```python
from build123d import *

# Parameters (mm, degrees)
BOSS_EXTRUDE1_DEPTH = 30
CUT_EXTRUDE2_REACH  = 61.852
SKETCH3_R           = 2
SKETCH3_R_2         = 6
FILLET1_R           = 1


with BuildPart() as part:
    # Sketch2 → Boss-Extrude1 (new body)
    with BuildSketch(Plane(origin=(0, 0, 0), x_dir=(1, 0, 0), z_dir=(0, 1, 0))):
        with BuildLine():
            Line((0, 50), (13.5, 50))
            Line((13.5, 50), (13.5, 0))
            Line((13.5, 0), (8.5, 0))
            Line((8.5, 0), (8.5, 25))
            ThreePointArc((8.5, 25), (7.621320344, 27.121320344), (5.5, 28))
            Line((5.5, 28), (0, 28))
            Line((0, 28), (0, 33))
            ThreePointArc((0, 33), (6, 39), (0, 45))
            Line((0, 45), (0, 50))
        make_face()
    extrude(amount=BOSS_EXTRUDE1_DEPTH)

    # Sketch3 → Cut-Extrude2 (cut, up to next)
    with BuildSketch(Plane(origin=(13.5, 0, 0), x_dir=(0, 0, -1), z_dir=(1, 0, 0)), mode=Mode.PRIVATE) as cut_extrude2_sk1:
        with BuildLine():
            ThreePointArc((0, 15), (3.514718626, 23.485281374), (12, 27))
            Line((12, 27), (22, 30))
            Line((22, 30), (0, 30))
            Line((0, 30), (0, 15))
        make_face()
    cut_extrude2_tool1 = extrude(cut_extrude2_sk1.sketch, amount=-CUT_EXTRUDE2_REACH, mode=Mode.PRIVATE) & part.part
    # Sketch3 → Cut-Extrude2 (cut, up to next)
    with BuildSketch(Plane(origin=(13.5, 0, 0), x_dir=(0, 0, -1), z_dir=(1, 0, 0)), mode=Mode.PRIVATE) as cut_extrude2_sk2:
        with BuildLine():
            ThreePointArc((12, 3), (3.514718626, 6.514718626), (0, 15))
            Line((0, 15), (0, 0))
            Line((0, 0), (22, 0))
            Line((22, 0), (12, 3))
        make_face()
    cut_extrude2_tool2 = extrude(cut_extrude2_sk2.sketch, amount=-CUT_EXTRUDE2_REACH, mode=Mode.PRIVATE) & part.part
    # Sketch3 → Cut-Extrude2 (cut, up to next)
    with BuildSketch(Plane(origin=(13.5, 0, 0), x_dir=(0, 0, -1), z_dir=(1, 0, 0)), mode=Mode.PRIVATE) as cut_extrude2_sk3:
        with Locations((30.5, 5)):
            Circle(SKETCH3_R)
    cut_extrude2_tool3 = extrude(cut_extrude2_sk3.sketch, amount=-CUT_EXTRUDE2_REACH, mode=Mode.PRIVATE) & part.part
    # Sketch3 → Cut-Extrude2 (cut, up to next)
    with BuildSketch(Plane(origin=(13.5, 0, 0), x_dir=(0, 0, -1), z_dir=(1, 0, 0)), mode=Mode.PRIVATE) as cut_extrude2_sk4:
        with Locations((47.5, 5)):
            Circle(SKETCH3_R)
    cut_extrude2_tool4 = extrude(cut_extrude2_sk4.sketch, amount=-CUT_EXTRUDE2_REACH, mode=Mode.PRIVATE) & part.part
    # Sketch3 → Cut-Extrude2 (cut, up to next)
    with BuildSketch(Plane(origin=(13.5, 0, 0), x_dir=(0, 0, -1), z_dir=(1, 0, 0)), mode=Mode.PRIVATE) as cut_extrude2_sk5:
        with Locations((47.5, 5)):
            Circle(SKETCH3_R)
    cut_extrude2_tool5 = extrude(cut_extrude2_sk5.sketch, amount=-CUT_EXTRUDE2_REACH, mode=Mode.PRIVATE) & part.part
    # Sketch3 → Cut-Extrude2 (cut, up to next)
    with BuildSketch(Plane(origin=(13.5, 0, 0), x_dir=(0, 0, -1), z_dir=(1, 0, 0)), mode=Mode.PRIVATE) as cut_extrude2_sk6:
        with Locations((12, 15)):
            Circle(SKETCH3_R_2)
    cut_extrude2_tool6 = extrude(cut_extrude2_sk6.sketch, amount=-CUT_EXTRUDE2_REACH, mode=Mode.PRIVATE) & part.part
    # Sketch3 → Cut-Extrude2 (cut, up to next)
    with BuildSketch(Plane(origin=(13.5, 0, 0), x_dir=(0, 0, -1), z_dir=(1, 0, 0)), mode=Mode.PRIVATE) as cut_extrude2_sk7:
        with Locations((30.5, 25)):
            Circle(SKETCH3_R)
    cut_extrude2_tool7 = extrude(cut_extrude2_sk7.sketch, amount=-CUT_EXTRUDE2_REACH, mode=Mode.PRIVATE) & part.part
    # Sketch3 → Cut-Extrude2 (cut, up to next)
    with BuildSketch(Plane(origin=(13.5, 0, 0), x_dir=(0, 0, -1), z_dir=(1, 0, 0)), mode=Mode.PRIVATE) as cut_extrude2_sk8:
        with Locations((47.5, 25)):
            Circle(SKETCH3_R)
    cut_extrude2_tool8 = extrude(cut_extrude2_sk8.sketch, amount=-CUT_EXTRUDE2_REACH, mode=Mode.PRIVATE) & part.part
    add(cut_extrude2_tool1.solids().sort_by_distance((13.5, 27.014261, -6.456835))[0], mode=Mode.SUBTRACT)
    add(cut_extrude2_tool2.solids().sort_by_distance((13.5, 2.985739, -6.456835))[0], mode=Mode.SUBTRACT)
    add(cut_extrude2_tool3.solids().sort_by_distance((13.5, 5, -30.5))[0], mode=Mode.SUBTRACT)
    add(cut_extrude2_tool4.solids().sort_by_distance((13.5, 5, -47.5))[0], mode=Mode.SUBTRACT)
    add(cut_extrude2_tool5.solids().sort_by_distance((13.5, 5, -47.5))[0], mode=Mode.SUBTRACT)
    add(cut_extrude2_tool6.solids().sort_by_distance((13.5, 15, -12))[0], mode=Mode.SUBTRACT)
    add(cut_extrude2_tool7.solids().sort_by_distance((13.5, 25, -30.5))[0], mode=Mode.SUBTRACT)
    add(cut_extrude2_tool8.solids().sort_by_distance((13.5, 25, -47.5))[0], mode=Mode.SUBTRACT)

    # Fillet1
    fillet1_edges = [part.edges().sort_by_distance(p)[0] for p in [
        (13.5, 15, -6),
        (8.5, 15, -6),
    ]]
    fillet(fillet1_edges, radius=FILLET1_R)


solid = part.part
```
Design review of the part built by this model. Coordinates are the model's own, in mm. A direction names the side the tool comes from. Round coordinates to 2 decimals unless told otherwise and drop trailing zeros. Order: outer loops, then holes, each group sorted by start corner. A loop starts at its lowest first (then second) coordinate and runs counter-clockwise, first axis right, second up. Notation, with made-up numbers: (64.25, 22) - (83.25, 22) arc R26 ccw to (83.25, 46) - close; hole circle Ø7 at (33, 25.5). An arc over 180 degrees is marked (long way). One line per question, with ' | ' between items.
Item 1: Take a section at B-B, the plane x = 3.75. Write out the cut boundary in (y, z).
Checks:
outline: (0, -50) - (30, -50) - (30, -43.68) - (0, -43.68) - close; (0, -34.32) - (30, -34.32) - (30, -28) - (0, -28) - close; hole circle Ø4 at (5, -47.5); hole circle Ø4 at (5, -30.5); hole circle Ø4 at (25, -47.5); hole circle Ø4 at (25, -30.5)
Item 2: Take a section at C-C, the plane y = 5. Write out the cut boundary in (x, z).
Checks:
outline: (0, -50) - (13.5, -50) - (13.5, -49.5) - (0, -49.5) - close; (0, -45.5) - (13.5, -45.5) - (13.5, -32.5) - (0, -32.5) - (0, -33) arc R6 cw to (0, -45) - close; (0, -28.5) - (13.5, -28.5) - (13.5, -5.37) - (8.5, -5.37) - (8.5, -25) arc R3 cw to (5.5, -28) - (0, -28) - close
Item 3: Wall thickness on line 1 (Y direction, x = 4.5, z = -47.5); line 2 (Y direction, x = 11, z = -47); line 3 (Z direction, x = 12.25, y = 6): over which ranges is each line inside the solid? List them lowest first. Write a range as [from, to].
Checks:
line 1: [0, 3], [7, 23], [27, 30] | line 2: [0, 3.06], [6.94, 23.06], [26.94, 30] | line 3: [-50, -49.23], [-45.77, -32.23], [-28.77, -4.06]
Item 4: Machinability: for faces 4 (the face through (8.5, 15, -21)), 5 (the face through (11.02, 12.7, -17.54)), which of the approach directions +Z, -Z, +X, -X, +Y, -Y give a long, thin tool a straight path to every point of the face, cutting with its end or side? Answer none if there is none.
Checks:
face 4: +Z, -X, +Y, -Y | face 5: +X, -X
Item 5: Draft analysis for pull direction Z (two halves, no side actions). For faces 1 (the face through (11.04, 28.48, -16.93)), 2 (the face through (6.844, 5.088, -45.502)), 3 (the face through (7, 15, -50)), state which applies: +Z half, -Z half, draft (parallel to the pull), parting line (faces both ways), or undercut.
Checks:
face 1: +Z half | face 2: undercut | face 3: -Z half
Item 6: Take a section at D-D, the plane y = 27.75. Write out the cut boundary in (x, z), then the cut area to 3 significant figures.
Checks:
outline: (0, -50) - (13.5, -50) - (13.5, -14.5) - (8.5, -14.5) - (8.5, -25) arc R3 cw to (5.5, -28) - (0, -28) - (0, -33) arc R6 cw to (0, -45) - close | area: 310 mm²
Item 7: For P1, Ø15.5, axis at y = 15, z = -12, coming from the -X side; P2, Ø4, axis at x = 12, z = -19, coming from the +Y side; P3, Ø8, axis at x = 1.5, y = 11.5, coming from the +Z side; P4, Ø3.5, axis at y = 25, z = -47.5, coming from the +X side, all flat-tipped, find the tip position at first contact; note any pin that passes through.
Checks:
P1: x = 8.5 | P2: y = 29.7 | P3: z = -28 | P4: through
Item 8: Take a section at A-A, the plane z = -30.5. Write out the cut boundary in (x, y).
Checks:
outline: (0, 0) - (13.5, 0) - (13.5, 3) - (0, 3) - close; (0, 7) - (13.5, 7) - (13.5, 23) - (0, 23) - close; (0, 27) - (13.5, 27) - (13.5, 30) - (0, 30) - close
